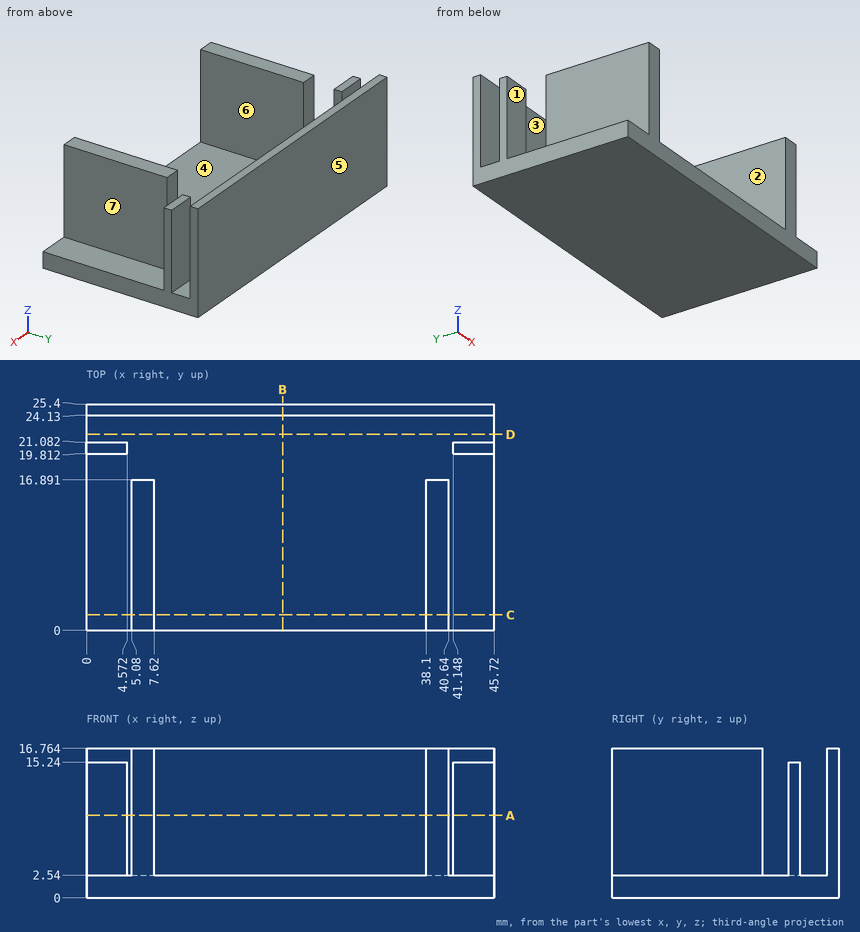
The drawing under review shows one solid part. Ordinate dimensions are in mm from its lowest x, y, z. A direction names the side the tool comes from. Round coordinates to 2 decimals unless told otherwise and drop trailing zeros. Write each loop counter-clockwise with the first axis right and the second up, starting at its lowest first coordinate (ties: lowest second). Pieces come first, ordered by that corner, then holes. Notation, with made-up numbers: (5, 67) - (56, 67) arc R19 cw to (56, 103) - close; hole circle Ø1 at (11, 55). An arc over 180 degrees is marked (long way). One line per question, with ' | ' between items.
Item 1: Add section B-B, the plane x = 22. Give the boundary of the cut face in (y, z), then the cut area to 3 significant figures.
Resolved:
outline: (0, 0) - (25.4, 0) - (25.4, 16.76) - (24.13, 16.76) - (24.13, 2.54) - (0, 2.54) - close | area: 82.6 mm2
Item 2: For P1, Ø8, axis at y = 10, z = 8.5, coming from the +X side; P2, Ø12, axis at x = 5.5, y = 17.5, coming from the +Z side; P3, Ø1.4, axis at x = 2.5, y = 20.5, coming from the +Z side; P4, Ø4, axis at y = 14, z = 7, coming from the -X side, all flat-tipped, find the tip position at first contact; note any pin that passes through.
Resolved:
P1: stops at x = 40.64 | P2: stops at z = 16.76 | P3: stops at z = 15.24 | P4: stops at x = 5.08
Item 3: Add section D-D, the plane y = 22. Give the boundary of the cut face in (x, z), then the cut area to 3 significant figures.
Resolved:
outline: (0, 0) - (45.72, 0) - (45.72, 2.54) - (0, 2.54) - close | area: 116 mm2
Item 4: Add section C-C, the plane y = 1.75. Give the boundary of the cut face in (x, z).
Resolved:
outline: (0, 0) - (45.72, 0) - (45.72, 2.54) - (40.64, 2.54) - (40.64, 16.76) - (38.1, 16.76) - (38.1, 2.54) - (7.62, 2.54) - (7.62, 16.76) - (5.08, 16.76) - (5.08, 2.54) - (0, 2.54) - close
Item 5: Add section A-A, the plane z = 9.25. Give the boundary of the cut face in (x, y), then the cut area to 3 significant figures.
Resolved:
outline: (0, 19.81) - (4.57, 19.81) - (4.57, 21.08) - (0, 21.08) - close; (0, 24.13) - (45.72, 24.13) - (45.72, 25.4) - (0, 25.4) - close; (5.08, 0) - (7.62, 0) - (7.62, 16.89) - (5.08, 16.89) - close; (38.1, 0) - (40.64, 0) - (40.64, 16.89) - (38.1, 16.89) - close; (41.15, 19.81) - (45.72, 19.81) - (45.72, 21.08) - (41.15, 21.08) - close | area: 155 mm2
Item 6: The part is to be moulded in two halves that separate along X. For the marked faces 4, 5, 6 and 7, say which applies: pulls with the +X half, pulls with the -X half, needs draft (parallel to the pull), parting line crosses it, or undercut.
Resolved:
face 4: undercut | face 5: needs draft | face 6: undercut | face 7: pulls with the +X half
Item 7: For the marked faces 1, 2 and 3, list the 3-axis set-ups (+Z, -Z, +X, -X, +Y, -Y) from which the entire face can be reached by the end or side of a thin tool; tool diameter is ignored.
Resolved:
face 1: +Z, +X, -X, -Y | face 2: +Z, -Y | face 3: +Z, +X, -X
Item 8: To check wall thickness, follow probe 1 along X at (y, z) = (6.25, 11.25); probe 2 along Y at (x, z) = (40, 2.75); probe 3 along X at (y, z) = (20, 5.75). State the ranges of each line that lie inside material, in increasing order.
Resolved:
probe 1: x = 5.08 to 7.62, 38.1 to 40.64 | probe 2: y = 0 to 16.89, 24.13 to 25.4 | probe 3: x = 0 to 4.57, 41.15 to 45.72
